```python
from build123d import *

# Parameters (mm, degrees)
SKETCH1_W             = 7
SKETCH1_H             = 5
BOSS_EXTRUDE1_DEPTH   = 5
CUT_EXTRUDE1_DEPTH    = 7
SKETCH4_R             = 1.5
BOSS_EXTRUDE3_DEPTH   = 14
F_1_5MM_DOWEL_HOLE2_D = 1.5


with BuildPart() as part:
    # Sketch1 → Boss-Extrude1 (new body)
    with BuildSketch(Plane.XY):
        with Locations((-1.19986884, 2.172533045)):
            Rectangle(SKETCH1_W, SKETCH1_H)
    extrude(amount=BOSS_EXTRUDE1_DEPTH)

    # Sketch2 → Cut-Extrude1 (cut)
    with BuildSketch(Plane.ZY.offset(4.69986884)):
        with BuildLine():
            Line((2.5, 4.672533045), (0, 4.672533045))
            Line((0, 4.672533045), (0, 0.672533045))
            add(Edge.make_bspline(
                [(0, 0.672533045), (2.331009943, 2.039673482), (2.5, 4.672533045)],
                knots=[0, 0, 0, 1, 1, 1], degree=2))
        make_face()
    extrude(amount=-CUT_EXTRUDE1_DEPTH, mode=Mode.SUBTRACT)

    # Sketch4 → Boss-Extrude3 (add)
    with BuildSketch(Plane.XZ.offset(0.327466955)):
        with Locations((-1.19986884, 2)):
            Circle(SKETCH4_R)
    extrude(amount=BOSS_EXTRUDE3_DEPTH)

    # Ø1.5mm Dowel Hole2 (through all)
    with Locations(Plane.ZY.offset(4.69986884)):
        with Locations((2, -12.327466955)):
            Hole(F_1_5MM_DOWEL_HOLE2_D / 2)


solid = part.part
```
The listing builds one solid part. Answer for the finished solid, in the listing's coordinates (mm). Coordinates: 2 decimals unless noted, no trailing zeros. Order: outer loops, then holes, each group sorted by start corner. A loop starts at its lowest first (then second) coordinate and runs counter-clockwise, first axis right, second up. Notation, with made-up numbers: M -30,67 L -6,67 A11 ccw -6,73 Z; hole C -13,7.5 d3. An arc over 180 degrees is marked long. Answer as a JSON object with one key per item and string values. Group by question number.
1. Flat-ended cylindrical pins translate along their axes: P1, Ø3, axis at x = -3.5, y = -8, coming from the +Z side; P2, Ø1.5, axis at x = -3, z = 4.5, coming from the -Y side; P3, Ø3, axis at y = -9, z = 3, coming from the -X side. Find the tip coordinate at first contact, or state that the pin passes through.
2. Section B-B on z = 4.7 is taken. Write down the section's boundary in (x, y).
3. Straight lines are drawn through the part: line 1 (Y direction, x = -4, z = 4); line 2 (Y direction, x = -2.25, z = 1.65); line 3 (Y direction, x = -2, z = 2). For each, find the intervals that lie inside material, in ascending order.
4. Section A-A on y = -5.25 is taken. Write down the section's boundary in (x, z), then the cut area to 3 significant figures.
5. Determine the mould class of faces 1 (the flat face through (-1, -14.327, 2)), 2 (the flat face through (-1, 2, 5)), 3 (the cylindrical face through (-1.179, -12.102, 1.285)), 4 (the cylindrical face through (-2.7, -7.23, 2.07)) for opening direction Z: released by +Z, released by -Z, zero draft, split by the parting line, or undercut.
Values follow:
{
 "1": {"P1": "z = 3.27", "P2": "y = -0.33", "P3": "x = -2.7"},
 "2": {"outline": "M -4.7,-0.33 L 2.3,-0.33 L 2.3,4.67 L -4.7,4.67 Z"},
 "3": {"line 1": "-0.33 to 4.67", "line 2": "-14.33 to -12.99, -11.66 to 2.14", "line 3": "-14.33 to -13.08, -11.58 to 2.73"},
 "4": {"outline": "C -1.2,2 d3", "area": "7.07 mm2"},
 "5": {"face 1": "zero draft", "face 2": "released by +Z", "face 3": "undercut", "face 4": "split by the parting line"}
}
